Can you work these out from the model? Positions are in its coordinate system, mm. Give positions to 0.01 mm unless a question says otherwise; leave off trailing zeros. Order: outer loops, then holes, each group sorted by start corner. A loop starts at its lowest first (then second) coordinate and runs counter-clockwise, first axis right, second up. Notation, with made-up numbers: M -7,78.25 L 50,78.25 A33 cw 50,111.25 Z; hole C 40.5,48.5 d7. An arc over 180 degrees is marked long. Answer as a JSON object with one key per item and string values.
```python
from build123d import *

# Parameters (mm, degrees)
SKETCH1_W           = 220
SKETCH1_H           = 600
SKETCH1_R           = 2.1
SKETCH1_R_2         = 1.6
SKETCH1_W_2         = 100
SKETCH1_H_2         = 320
BOSS_EXTRUDE1_DEPTH = 3.175
FILLET1_R           = 3.2


with BuildPart() as part:
    # Sketch1 → Boss-Extrude1 (new body)
    with BuildSketch(Plane(origin=(0, 0, 0), x_dir=(1, 0, 0), z_dir=(0, 1, 0))):
        Rectangle(SKETCH1_W, SKETCH1_H)
        with Locations(Location((100, 290, 0), (0, 0, 270))):
            Circle(SKETCH1_R, mode=Mode.SUBTRACT)
        with Locations(Location((100, 232, 0), (0, 0, 270))):
            Circle(SKETCH1_R, mode=Mode.SUBTRACT)
        with Locations(Location((100, 174, 0), (0, 0, 270))):
            Circle(SKETCH1_R, mode=Mode.SUBTRACT)
        with Locations(Location((100, 116, 0), (0, 0, 270))):
            Circle(SKETCH1_R, mode=Mode.SUBTRACT)
        with Locations(Location((100, 58, 0), (0, 0, 270))):
            Circle(SKETCH1_R, mode=Mode.SUBTRACT)
        with Locations(Location((100, 0, 0), (0, 0, 270))):
            Circle(SKETCH1_R, mode=Mode.SUBTRACT)
        with Locations(Location((100, -58, 0), (0, 0, 270))):
            Circle(SKETCH1_R, mode=Mode.SUBTRACT)
        with Locations(Location((100, -116, 0), (0, 0, 270))):
            Circle(SKETCH1_R, mode=Mode.SUBTRACT)
        with Locations(Location((100, -174, 0), (0, 0, 270))):
            Circle(SKETCH1_R, mode=Mode.SUBTRACT)
        with Locations(Location((100, -232, 0), (0, 0, 270))):
            Circle(SKETCH1_R, mode=Mode.SUBTRACT)
        with Locations(Location((100, -290, 0), (0, 0, 270))):
            Circle(SKETCH1_R, mode=Mode.SUBTRACT)
        with Locations(Location((84, -232, 0), (0, 0, 90))):
            Circle(SKETCH1_R, mode=Mode.SUBTRACT)
        with Locations(Location((84, -174, 0), (0, 0, 90))):
            Circle(SKETCH1_R, mode=Mode.SUBTRACT)
        with Locations(Location((84, -116, 0), (0, 0, 90))):
            Circle(SKETCH1_R, mode=Mode.SUBTRACT)
        with Locations(Location((84, -58, 0), (0, 0, 90))):
            Circle(SKETCH1_R, mode=Mode.SUBTRACT)
        with Locations(Location((84, 0, 0), (0, 0, 90))):
            Circle(SKETCH1_R, mode=Mode.SUBTRACT)
        with Locations(Location((84, 58, 0), (0, 0, 90))):
            Circle(SKETCH1_R, mode=Mode.SUBTRACT)
        with Locations(Location((84, 116, 0), (0, 0, 90))):
            Circle(SKETCH1_R, mode=Mode.SUBTRACT)
        with Locations(Location((84, 174, 0), (0, 0, 90))):
            Circle(SKETCH1_R, mode=Mode.SUBTRACT)
        with Locations(Location((84, 232, 0), (0, 0, 90))):
            Circle(SKETCH1_R, mode=Mode.SUBTRACT)
        with Locations(Location((84, 290, 0), (0, 0, 90))):
            Circle(SKETCH1_R, mode=Mode.SUBTRACT)
        with Locations(Location((92, 0, 0), (0, 0, 270))):
            Circle(SKETCH1_R_2, mode=Mode.SUBTRACT)
        with Locations(Location((92, 235, 0), (0, 0, 270))):
            Circle(SKETCH1_R_2, mode=Mode.SUBTRACT)
        with Locations(Location((92, -235, 0), (0, 0, 90))):
            Circle(SKETCH1_R_2, mode=Mode.SUBTRACT)
        with Locations(Location((-92, 235, 0), (0, 0, 90))):
            Circle(SKETCH1_R_2, mode=Mode.SUBTRACT)
        with Locations(Location((-84, 290, 0), (0, 0, 270))):
            Circle(SKETCH1_R, mode=Mode.SUBTRACT)
        with Locations(Location((-84, 232, 0), (0, 0, 270))):
            Circle(SKETCH1_R, mode=Mode.SUBTRACT)
        with Locations(Location((-84, 174, 0), (0, 0, 270))):
            Circle(SKETCH1_R, mode=Mode.SUBTRACT)
        with Locations(Location((-84, 116, 0), (0, 0, 270))):
            Circle(SKETCH1_R, mode=Mode.SUBTRACT)
        with Locations(Location((-100, 116, 0), (0, 0, 90))):
            Circle(SKETCH1_R, mode=Mode.SUBTRACT)
        with Locations(Location((-100, 174, 0), (0, 0, 90))):
            Circle(SKETCH1_R, mode=Mode.SUBTRACT)
        with Locations(Location((-100, 232, 0), (0, 0, 90))):
            Circle(SKETCH1_R, mode=Mode.SUBTRACT)
        with Locations(Location((-100, 290, 0), (0, 0, 90))):
            Circle(SKETCH1_R, mode=Mode.SUBTRACT)
        with Locations(Location((-92, -235, 0), (0, 0, 270))):
            Circle(SKETCH1_R_2, mode=Mode.SUBTRACT)
        with Locations(Location((-92, 0, 0), (0, 0, 90))):
            Circle(SKETCH1_R_2, mode=Mode.SUBTRACT)
        with Locations(Location((-84, 58, 0), (0, 0, 270))):
            Circle(SKETCH1_R, mode=Mode.SUBTRACT)
        with Locations(Location((-84, 0, 0), (0, 0, 270))):
            Circle(SKETCH1_R, mode=Mode.SUBTRACT)
        with Locations(Location((-84, -58, 0), (0, 0, 270))):
            Circle(SKETCH1_R, mode=Mode.SUBTRACT)
        with Locations(Location((-84, -116, 0), (0, 0, 270))):
            Circle(SKETCH1_R, mode=Mode.SUBTRACT)
        with Locations(Location((-84, -174, 0), (0, 0, 270))):
            Circle(SKETCH1_R, mode=Mode.SUBTRACT)
        with Locations(Location((-84, -232, 0), (0, 0, 270))):
            Circle(SKETCH1_R, mode=Mode.SUBTRACT)
        with Locations(Location((-100, -290, 0), (0, 0, 90))):
            Circle(SKETCH1_R, mode=Mode.SUBTRACT)
        with Locations(Location((-100, -232, 0), (0, 0, 90))):
            Circle(SKETCH1_R, mode=Mode.SUBTRACT)
        with Locations(Location((-100, -174, 0), (0, 0, 90))):
            Circle(SKETCH1_R, mode=Mode.SUBTRACT)
        with Locations(Location((-100, -116, 0), (0, 0, 90))):
            Circle(SKETCH1_R, mode=Mode.SUBTRACT)
        with Locations(Location((-100, -58, 0), (0, 0, 90))):
            Circle(SKETCH1_R, mode=Mode.SUBTRACT)
        with Locations(Location((-100, 0, 0), (0, 0, 90))):
            Circle(SKETCH1_R, mode=Mode.SUBTRACT)
        with Locations(Location((-100, 58, 0), (0, 0, 90))):
            Circle(SKETCH1_R, mode=Mode.SUBTRACT)
        with Locations(Location((56, 290, 0), (0, 0, 90))):
            Circle(SKETCH1_R, mode=Mode.SUBTRACT)
        with Locations(Location((28, 290, 0), (0, 0, 90))):
            Circle(SKETCH1_R, mode=Mode.SUBTRACT)
        with Locations(Location((0, 290, 0), (0, 0, 90))):
            Circle(SKETCH1_R, mode=Mode.SUBTRACT)
        with Locations(Location((-28, 290, 0), (0, 0, 90))):
            Circle(SKETCH1_R, mode=Mode.SUBTRACT)
        with Locations(Location((-56, 290, 0), (0, 0, 90))):
            Circle(SKETCH1_R, mode=Mode.SUBTRACT)
        with Locations(Location((56, 232, 0), (0, 0, 90))):
            Circle(SKETCH1_R, mode=Mode.SUBTRACT)
        with Locations(Location((28, 232, 0), (0, 0, 90))):
            Circle(SKETCH1_R, mode=Mode.SUBTRACT)
        with Locations(Location((0, 232, 0), (0, 0, 90))):
            Circle(SKETCH1_R, mode=Mode.SUBTRACT)
        with Locations(Location((-28, 232, 0), (0, 0, 90))):
            Circle(SKETCH1_R, mode=Mode.SUBTRACT)
        with Locations(Location((-56, 232, 0), (0, 0, 90))):
            Circle(SKETCH1_R, mode=Mode.SUBTRACT)
        with Locations(Location((85, -290, 0), (0, 0, 270))):
            Circle(SKETCH1_R, mode=Mode.SUBTRACT)
        with Locations(Location((85, -268, 0), (0, 0, 90))):
            Circle(SKETCH1_R, mode=Mode.SUBTRACT)
        with Locations(Location((100, -268, 0), (0, 0, 90))):
            Circle(SKETCH1_R, mode=Mode.SUBTRACT)
        with Locations(Location((-85, -290, 0), (0, 0, 90))):
            Circle(SKETCH1_R, mode=Mode.SUBTRACT)
        with Locations(Location((-100, -268, 0), (0, 0, 270))):
            Circle(SKETCH1_R, mode=Mode.SUBTRACT)
        with Locations(Location((-85, -268, 0), (0, 0, 270))):
            Circle(SKETCH1_R, mode=Mode.SUBTRACT)
        with Locations(Location((17, -251, 0), (0, 0, 270))):
            Circle(SKETCH1_R, mode=Mode.SUBTRACT)
        with Locations(Location((7, -251, 0), (0, 0, 270))):
            Circle(SKETCH1_R, mode=Mode.SUBTRACT)
        with Locations(Location((17, -211, 0), (0, 0, 90))):
            Circle(SKETCH1_R, mode=Mode.SUBTRACT)
        with Locations(Location((7, -211, 0), (0, 0, 90))):
            Circle(SKETCH1_R, mode=Mode.SUBTRACT)
        with Locations((0, 40)):
            Rectangle(SKETCH1_W_2, SKETCH1_H_2, mode=Mode.SUBTRACT)
    extrude(amount=BOSS_EXTRUDE1_DEPTH)

    # Fillet1
    fillet1_edges = [part.edges().sort_by_distance(p)[0] for p in [
        (110, 1.5875, 300),
        (-110, 1.5875, 300),
        (-110, 1.5875, -300),
        (110, 1.5875, -300),
    ]]
    fillet(fillet1_edges, radius=FILLET1_R)


solid = part.part
```
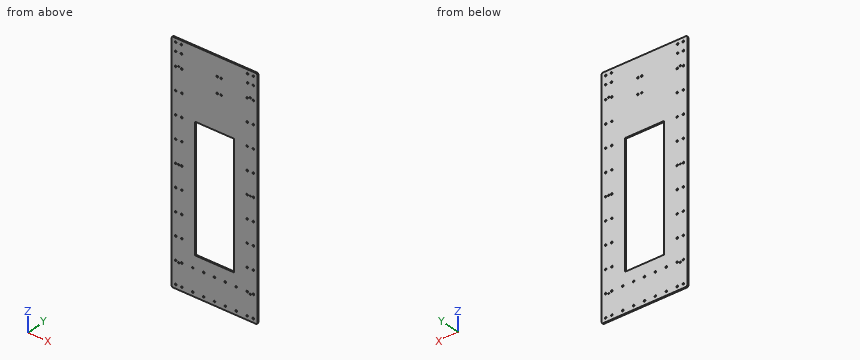
1) I want a section at C-C on y = 2. Count the separate pieces of the cut face and the enclosed holes in it, and give its area (3 significant figures).
Results found:
{"separate pieces": "1", "enclosed holes": "69", "area": "99,100 mm²"}
2) I want a section at A-A on x = -42.5. Write out the boundary of the cut face in (y, z) (3 decimals), and give its area (3 significant figures).
Results found:
{"outline": "M 0,-300 L 3.175,-300 L 3.175,-200 L 0,-200 Z; M 0,120 L 3.175,120 L 3.175,300 L 0,300 Z", "area": "889 mm²"}
3) I'm going to push a flat-ended pin straight in: pin 1 Ø4 at (x, z) = (7, 251) entering from +Y. Where does the tip first touch, or does it pass through?
Results found:
{"pin 1": "passes through"}
4) I need wall thicknesses on L1, parallel to Z at x = 56.5, y = 2.8; L2, parallel to X at y = 2.3, z = 174; L3, parallel to Z at x = -92, y = 1.2. Which ranges of each line are inside material? Lowest first, please.
Results found:
{"L1": "z = -300 to -292.04, -287.96 to -234.04, -229.96 to 300", "L2": "x = -110 to -102.1, -97.9 to -86.1, -81.9 to 81.9, 86.1 to 97.9, 102.1 to 110", "L3": "z = -300 to -236.6, -233.4 to -1.6, 1.6 to 233.4, 236.6 to 300"}
5) I want a section at B-B on z = -147.5. Write out the boundary of the cut face in (x, y) (3 decimals), and give its area (3 significant figures).
Results found:
{"outline": "M -110,0 L -50,0 L -50,3.175 L -110,3.175 Z; M 50,0 L 110,0 L 110,3.175 L 50,3.175 Z", "area": "381 mm²"}
